from build123d import *

# Parameters (mm, degrees)
F0_W          = 100
F0_H          = 40
F1_DEPTH      = 10
F3_DEPTH      = 10
F4_W          = 40.0635205954
F4_H          = 3
F5_DEPTH      = 40.001
F6_R          = 2.25
F7_DEPTH      = 10.001
F8_R          = 4.5
F10_DEPTH     = 5.7
F11_T1_DEPTH  = 45.7
F11_T3_DEPTH  = 45.7
F11_T5_DEPTH  = 50
F11_T7_DEPTH  = 50
F11_T9_DEPTH  = 50
F11_T11_DEPTH = 50
F12_R         = 3


# Not quite as in the source:
# - a fillet or chamfer that OpenCascade refuses, or shapes differently, is made with other operations: its cross-section is extruded or revolved along the edge and cut away or added
# - the program builds the solid bodies; features that only make, move or delete a surface that nothing else refers to are left out


with BuildPart() as f1:
    # F0 (on Top) → F1 (new body)
    with BuildSketch(Plane.XY):
        with Locations((-50, 20)):
            Rectangle(F0_W, F0_H)
    extrude(amount=F1_DEPTH)

    # F2 (on face) → F3 (join)
    with BuildSketch(Plane.XZ):
        with BuildLine():
            ThreePointArc((-30, 35), (-50, 55), (-70, 35))
            Line((-70, 35), (-70, 0))
            Line((-70, 0), (-30, 0))
            Line((-30, 0), (-30, 35))
        make_face()
    extrude(amount=-F3_DEPTH)

    # F4 (on face) → F5 (cut, through all)
    with BuildSketch(Plane.XZ):
        with Locations((-49.9682397023, 1.5)):
            Rectangle(F4_W, F4_H)
    extrude(amount=-F5_DEPTH, mode=Mode.SUBTRACT)

    # F6 (on face) → F7 (cut, through all)
    with BuildSketch(Plane(origin=(0, 10, 0), x_dir=(-1, 0, 0), z_dir=(0, 1, 0))):
        with Locations((50, 35)):
            Circle(F6_R)
    extrude(amount=-F7_DEPTH, mode=Mode.SUBTRACT)

    # F8 (on face) → F10 (join)
    with BuildSketch(Plane.XZ):
        with BuildLine():
            Line((-100, 10), (-100, 0))
            Line((-100, 0), (-70, 0))
            Line((-70, 0), (-70, 3))
            Line((-70, 3), (-29.9364794046, 3))
            Line((-29.9364794046, 3), (-29.9364794046, 0))
            Line((-29.9364794046, 0), (0, 0))
            Line((0, 0), (0, 10))
            Line((0, 10), (-30, 10))
            Line((-30, 10), (-30, 35))
            ThreePointArc((-30, 35), (-50, 55), (-70, 35))
            Line((-70, 35), (-70, 10))
            Line((-70, 10), (-100, 10))
        make_face()
        with Locations((-50, 35)):
            Circle(F8_R, mode=Mode.SUBTRACT)
    extrude(amount=F10_DEPTH)

    # F11: fillet of radius 8 on 8 edges, made by hand

    # F11_s2 → F11_t1 (join)
    with BuildSketch(Plane.XZ.offset(-40)):
        with BuildLine():
            ThreePointArc((-29.9364794046, 0), (-32.7173757878, 2.2111025509), (-36.181477403, 3))
            Line((-36.181477403, 3), (-29.9364794046, 3))
            Line((-29.9364794046, 3), (-29.9364794046, 0))
        make_face()
    extrude(amount=F11_T1_DEPTH)

    # F11_s4 → F11_t3 (join)
    with BuildSketch(Plane.XZ.offset(-40)):
        with BuildLine():
            ThreePointArc((-70, 0), (-67.2191036167, 2.2111025509), (-63.7550020016, 3))
            Line((-63.7550020016, 3), (-70, 3))
            Line((-70, 3), (-70, 0))
        make_face()
    extrude(amount=F11_T3_DEPTH)

    # F11_s6 → F11_t5 (cut)
    with BuildSketch(Plane.XY.offset(-20)):
        with BuildLine():
            ThreePointArc((-92, -5.7), (-97.6568542495, -3.3568542495), (-100, 2.3))
            Line((-100, 2.3), (-100, -5.7))
            Line((-100, -5.7), (-92, -5.7))
        make_face()
    extrude(amount=F11_T5_DEPTH, mode=Mode.SUBTRACT)

    # F11_s8 → F11_t7 (cut)
    with BuildSketch(Plane.XY.offset(-20)):
        with BuildLine():
            ThreePointArc((-8, -5.7), (-2.3431457505, -3.3568542495), (0, 2.3))
            Line((0, 2.3), (0, -5.7))
            Line((0, -5.7), (-8, -5.7))
        make_face()
    extrude(amount=F11_T7_DEPTH, mode=Mode.SUBTRACT)

    # F11_s10 → F11_t9 (cut)
    with BuildSketch(Plane.XY.offset(-20)):
        with BuildLine():
            ThreePointArc((-8, 40), (-2.3431457505, 37.6568542495), (0, 32))
            Line((0, 32), (0, 40))
            Line((0, 40), (-8, 40))
        make_face()
    extrude(amount=F11_T9_DEPTH, mode=Mode.SUBTRACT)

    # F11_s12 → F11_t11 (cut)
    with BuildSketch(Plane.XY.offset(-20)):
        with BuildLine():
            ThreePointArc((-92, 40), (-97.6568542495, 37.6568542495), (-100, 32))
            Line((-100, 32), (-100, 40))
            Line((-100, 40), (-92, 40))
        make_face()
    extrude(amount=F11_T11_DEPTH, mode=Mode.SUBTRACT)

    # F12
    f12_edges = [f1.edges().sort_by_distance(p)[0] for p in [
        (-30, -5.7, 22.5),
        (-50, -5.7, 55),
        (-50, 10, 55),
        (-70, -5.7, 22.5),
        (-30, 10, 22.5),
        (-70, 10, 22.5),
    ]]
    fillet(f12_edges, radius=F12_R)


solid = f1.part
Can you work these out from the model? Positions are in its coordinate system, mm. A direction names the side the tool comes from. Coordinates: 2 decimals unless noted, no trailing zeros. Order: outer loops, then holes, each group sorted by start corner. A loop starts at its lowest first (then second) coordinate and runs counter-clockwise, first axis right, second up. Notation, with made-up numbers: (19, 86) - (74, 86) arc R28 ccw to (74, 106) - close; hole circle Ø7 at (70.25, 63.5). An arc over 180 degrees is marked (long way). Answer as a JSON object with one key per item and string values. Group by question number.
Q1. On a 3-axis mill with a long thin cutter (end or side, diameter ignored), from which of +Z, -Z, +X, -X, +Y, -Y can I reach the whole of each face in a straight line? I mean faces 5 (the face through (-50, 10, 31)), 6 (the face through (-70, 2, 23)), 7 (the face through (-32.67, 17.47, 2.19)), 8 (the face through (-30, 2, 22)). Say none if no direction works.
Q2. Imagine slicing it at A-A (x = -50). Please give me the cut outline in (y, z).
Q3. We'd pull the mould along X, two halves only. Please class faces 1 (the face through (-67.26, 17.47, 2.19)), 2 (the face through (0, 17, 5)), 3 (the face through (-48.34, 5.07, 36.52)), 4 (the face through (-49, 17, 10)): +X half, -X half, draft (parallel to the pull), parting line (faces both ways), or undercut.
Q4. Imagine slicing it at C-C (z = 11). Please give me the cut outline in (x, y).
Q5. I need wall thicknesses on line 1 (Z direction, x = -50, y = 3.25); line 2 (Z direction, x = -46, y = 21.5); line 3 (Y direction, x = -53.5, z = 45.5). Which ranges of each line are inside material? Lowest first, please. Write a range as from..to.
Q6. Will these pins go through, and if not, where does the flat tip stop? P1, Ø2.5, axis at x = -51, z = 34, coming from the -Y side; P2, Ø8, axis at x = -12, y = 34, coming from the +Z side; P3, Ø6, axis at y = 11.5, z = 22, coming from the +X side.
Q7. Imagine slicing it at D-D (x = -89). Please give me the cut outline in (y, z), and give its area (3 significant figures).
Q8. Imagine slicing it at B-B (y = 21.5). Please give me the cut outline in (x, z) (3 decimals).
Determined:
{
 "1": {"face 5": "+Z, +X, -X, +Y", "face 6": "+Z, -X, +Y, -Y", "face 7": "-Z, +Y, -Y", "face 8": "+Z, +X, +Y, -Y"},
 "2": {"outline": "(-5.7, 3) - (40, 3) - (40, 10) - (10, 10) - (10, 32.75) - (0, 32.75) - (0, 30.5) - (-5.7, 30.5) - close; (-5.7, 39.5) - (0, 39.5) - (0, 37.25) - (10, 37.25) - (10, 52) arc R3 ccw to (7, 55) - (-2.7, 55) arc R3 ccw to (-5.7, 52) - close"},
 "3": {"face 1": "undercut", "face 2": "+X half", "face 3": "undercut", "face 4": "draft"},
 "4": {"outline": "(-70, -2.7) arc R3 ccw to (-67, -5.7) - (-33, -5.7) arc R3 ccw to (-30, -2.7) - (-30, 7) arc R3 ccw to (-33, 10) - (-67, 10) arc R3 ccw to (-70, 7) - close"},
 "5": {"line 1": "z = 3..32.75, 37.25..55", "line 2": "z = 3..10", "line 3": "y = -5.7..10"},
 "6": {"P1": "stops at y = 0", "P2": "stops at z = 10", "P3": "stops at x = -30.4"},
 "7": {"outline": "(-5.7, 0) - (40, 0) - (40, 10) - (-5.7, 10) - close", "area": "457 mm2"},
 "8": {"outline": "(-100, 0) - (-70, 0) arc R8 cw to (-63.755, 3) - (-36.181, 3) arc R8 cw to (-29.936, 0) - (0, 0) - (0, 10) - (-100, 10) - close"}
}
